Source: CAD feature listing. Evaluate the final solid. Frame: model axes, mm. A direction names the side the tool comes from. Round coordinates to 2 decimals unless told otherwise and drop trailing zeros. Loops run counter-clockwise (first coordinate to the right, second up) from the corner with the lowest first, then second, coordinate; pieces in that order, holes last. Notation, with made-up numbers: M -33,-2.75 L -4,-2.75 A24 ccw -4,10.25 Z; hole C 27.5,50.5 d6. An arc over 180 degrees is marked long. One line per item, written item: value.
from build123d import *

# Parameters (mm, degrees)
F0_R     = 3.175
F0_W     = 0.7229064099
F0_H     = 4.7706251523
F1_DEPTH = 3.048


with BuildPart() as f1:
    # F0 (on Front) → F1 (new body)
    with BuildSketch(Plane.XZ):
        with BuildLine():
            ThreePointArc((-9.4502929642, 115.490625), (-0.596483242, 104.7936951058), (9.525, 114.3))
            ThreePointArc((9.525, 114.3), (9.5063048942, 114.896483242), (9.4502929642, 115.490625))
            ThreePointArc((9.4502929642, 115.490625), (0, 123.825), (-9.4502929642, 115.490625))
        make_face()
        with Locations((0, 114.3)):
            Circle(F0_R, mode=Mode.SUBTRACT)
        with BuildLine():
            ThreePointArc((9.4502929642, 115.490625), (9.5063048942, 114.896483242), (9.525, 114.3))
            ThreePointArc((9.525, 114.3), (-0.596483242, 104.7936951058), (-9.4502929642, 115.490625))
            Line((-9.4502929642, 115.490625), (-15.7504882737, 65.484375))
            ThreePointArc((-15.7504882737, 65.484375), (0, 79.375), (15.7504882737, 65.484375))
            Line((15.7504882737, 65.484375), (9.4502929642, 115.490625))
        make_face()
        with Locations((-3.175, 100.0252)):
            Circle(F0_R, mode=Mode.SUBTRACT)
        with BuildLine():
            ThreePointArc((15.875, 63.5), (15.8438414904, 64.4941387366), (15.7504882737, 65.484375))
            ThreePointArc((15.7504882737, 65.484375), (0, 79.375), (-15.7504882737, 65.484375))
            ThreePointArc((-15.7504882737, 65.484375), (-15.8737438155, 63.6997054867), (-15.7954255641, 61.9125))
            ThreePointArc((-15.7954255641, 61.9125), (0, 47.625), (15.7954255641, 61.9125))
            ThreePointArc((15.7954255641, 61.9125), (15.8550939106, 62.7052534459), (15.875, 63.5))
        make_face()
        with Locations((0, 63.5)):
            Circle(F0_R, mode=Mode.SUBTRACT)
        with BuildLine():
            ThreePointArc((15.7954255641, 61.9125), (0, 47.625), (-15.7954255641, 61.9125))
            Line((-15.7954255641, 61.9125), (-9.4772553384, -0.9525))
            ThreePointArc((-9.4772553384, -0.9525), (-0.4768479324, 9.5130563464), (9.525, 0))
            ThreePointArc((9.525, 0), (6.8544082857, -6.6138273378), (0.3401785714, -9.5189234444))
            Line((0.3401785714, -9.5189234444), (44.7334821429, -7.9324362036))
            ThreePointArc((44.7334821429, -7.9324362036), (36.5125, 0), (44.7334821429, 7.9324362036))
            Line((44.7334821429, 7.9324362036), (18.9676000005, 8.8532337108))
            ThreePointArc((18.9676000005, 8.8532337108), (13.2611998974, 11.5713591498), (11.3411865923, 17.5933818124))
            Line((11.3411865923, 17.5933818124), (15.7954255641, 61.9125))
        make_face()
        Polygon((-5.7888228126, 31.6815939556), (-6.5549086035, 31.6815939556), (-7.3474591762, 33.7054533268), (-9.8978284182, 33.7054533268), (-10.6806288082, 31.6815939556), (-11.43, 31.6815939556), (-8.9144528394, 38.0721423349), (-8.2918340239, 38.0721423349), align=None, mode=Mode.SUBTRACT)
        with BuildLine():
            Line((-1.0349122593, 31.6815939556), (-1.7578186693, 31.6815939556))
            Line((-1.7578186693, 31.6815939556), (-1.7578186693, 34.7682232513))
            add(Edge.make_bspline(
                [(-1.7578186693, 34.7682232513), (-1.7578186693, 35.3504484524), (-2.0231629296, 35.6380788447)],
                knots=[0, 0, 0, 1, 1, 1], degree=2))
            add(Edge.make_bspline(
                [(-2.0231629296, 35.6380788447), (-2.2885071899, 35.9257092371), (-2.8554106751, 35.9257092371)],
                knots=[0, 0, 0, 1, 1, 1], degree=2))
            add(Edge.make_bspline(
                [(-2.8554106751, 35.9257092371), (-3.6033889837, 35.9257092371), (-3.9516097977, 35.5210766512)],
                knots=[0, 0, 0, 1, 1, 1], degree=2))
            add(Edge.make_bspline(
                [(-3.9516097977, 35.5210766512), (-4.2998306117, 35.1164440653), (-4.2998306117, 34.184605167)],
                knots=[0, 0, 0, 1, 1, 1], degree=2))
            Line((-4.2998306117, 34.184605167), (-4.2998306117, 31.6815939556))
            Line((-4.2998306117, 31.6815939556), (-5.0227370217, 31.6815939556))
            Line((-5.0227370217, 31.6815939556), (-5.0227370217, 36.452219108))
            Line((-5.0227370217, 36.452219108), (-4.4349402876, 36.452219108))
            Line((-4.4349402876, 36.452219108), (-4.3179380941, 35.7989568608))
            Line((-4.3179380941, 35.7989568608), (-4.2831160127, 35.7989568608))
            add(Edge.make_bspline(
                [(-4.2831160127, 35.7989568608), (-4.0602546917, 36.1513563246), (-3.6598007555, 36.3456635389)],
                knots=[0, 0, 0, 1, 1, 1], degree=2))
            add(Edge.make_bspline(
                [(-3.6598007555, 36.3456635389), (-3.2593468194, 36.5399707531), (-2.76765903, 36.5399707531)],
                knots=[0, 0, 0, 1, 1, 1], degree=2))
            add(Edge.make_bspline(
                [(-2.76765903, 36.5399707531), (-1.9054642944, 36.5399707531), (-1.4701882769, 36.1241951011)],
                knots=[0, 0, 0, 1, 1, 1], degree=2))
            add(Edge.make_bspline(
                [(-1.4701882769, 36.1241951011), (-1.0349122593, 35.7084194492), (-1.0349122593, 34.7932951499)],
                knots=[0, 0, 0, 1, 1, 1], degree=2))
            Line((-1.0349122593, 34.7932951499), (-1.0349122593, 31.6815939556))
        make_face(mode=Mode.SUBTRACT)
        with Locations((0.8099616135, 34.0669065318)):
            Rectangle(F0_W, F0_H, mode=Mode.SUBTRACT)
        with BuildLine():
            add(Edge.make_bspline(
                [(0.5090988301, 37.3812722398), (0.3872215452, 37.5010601999), (0.3872215452, 37.7448147697)],
                knots=[0, 0, 0, 1, 1, 1], degree=2))
            add(Edge.make_bspline(
                [(0.3872215452, 37.7448147697), (0.3872215452, 37.9927479893), (0.5090988301, 38.1083572995)],
                knots=[0, 0, 0, 1, 1, 1], degree=2))
            add(Edge.make_bspline(
                [(0.5090988301, 38.1083572995), (0.630976115, 38.2239666098), (0.8148367049, 38.2239666098)],
                knots=[0, 0, 0, 1, 1, 1], degree=2))
            add(Edge.make_bspline(
                [(0.8148367049, 38.2239666098), (0.9889471119, 38.2239666098), (1.1150030466, 38.1062679747)],
                knots=[0, 0, 0, 1, 1, 1], degree=2))
            add(Edge.make_bspline(
                [(1.1150030466, 38.1062679747), (1.2410589812, 37.9885693395), (1.2410589812, 37.7448147697)],
                knots=[0, 0, 0, 1, 1, 1], degree=2))
            add(Edge.make_bspline(
                [(1.2410589812, 37.7448147697), (1.2410589812, 37.5010601999), (1.1150030466, 37.3812722398)],
                knots=[0, 0, 0, 1, 1, 1], degree=2))
            add(Edge.make_bspline(
                [(1.1150030466, 37.3812722398), (0.9889471119, 37.2614842798), (0.8148367049, 37.2614842798)],
                knots=[0, 0, 0, 1, 1, 1], degree=2))
            add(Edge.make_bspline(
                [(0.8148367049, 37.2614842798), (0.630976115, 37.2614842798), (0.5090988301, 37.3812722398)],
                knots=[0, 0, 0, 1, 1, 1], degree=2))
        make_face(mode=Mode.SUBTRACT)
        with BuildLine():
            Line((3.3833134292, 34.1233183037), (3.4181355106, 34.1233183037))
            add(Edge.make_bspline(
                [(3.4181355106, 34.1233183037), (3.6047818669, 34.3893590056), (3.9878247624, 34.8197599318)],
                knots=[0, 0, 0, 1, 1, 1], degree=2))
            Line((3.9878247624, 34.8197599318), (5.5283536437, 36.452219108))
            Line((5.5283536437, 36.452219108), (6.3863697295, 36.452219108))
            Line((6.3863697295, 36.452219108), (4.4530477699, 34.4200024372))
            Line((4.4530477699, 34.4200024372), (6.5214794053, 31.6815939556))
            Line((6.5214794053, 31.6815939556), (5.6467487204, 31.6815939556))
            Line((5.6467487204, 31.6815939556), (3.9613599805, 33.9366719474))
            Line((3.9613599805, 33.9366719474), (3.4181355106, 33.4658774068))
            Line((3.4181355106, 33.4658774068), (3.4181355106, 31.6815939556))
            Line((3.4181355106, 31.6815939556), (2.7035864002, 31.6815939556))
            Line((2.7035864002, 31.6815939556), (2.7035864002, 38.4551852303))
            Line((2.7035864002, 38.4551852303), (3.4181355106, 38.4551852303))
            Line((3.4181355106, 38.4551852303), (3.4181355106, 34.8629393127))
            add(Edge.make_bspline(
                [(3.4181355106, 34.8629393127), (3.4181355106, 34.6247562759), (3.3833134292, 34.1233183037)],
                knots=[0, 0, 0, 1, 1, 1], degree=2))
        make_face(mode=Mode.SUBTRACT)
        with BuildLine():
            Line((10.8519534487, 31.6815939556), (10.3156933951, 31.6815939556))
            Line((10.3156933951, 31.6815939556), (10.1722264197, 32.3613209846))
            Line((10.1722264197, 32.3613209846), (10.1374043383, 32.3613209846))
            add(Edge.make_bspline(
                [(10.1374043383, 32.3613209846), (9.7808262247, 31.9128125762), (9.426337436, 31.7533274433)],
                knots=[0, 0, 0, 1, 1, 1], degree=2))
            add(Edge.make_bspline(
                [(9.426337436, 31.7533274433), (9.0718486473, 31.5938423105), (8.5397672435, 31.5938423105)],
                knots=[0, 0, 0, 1, 1, 1], degree=2))
            add(Edge.make_bspline(
                [(8.5397672435, 31.5938423105), (7.8307896661, 31.5938423105), (7.4282464051, 31.9601706069)],
                knots=[0, 0, 0, 1, 1, 1], degree=2))
            add(Edge.make_bspline(
                [(7.4282464051, 31.9601706069), (7.025703144, 32.3264989032), (7.025703144, 33.0006543992)],
                knots=[0, 0, 0, 1, 1, 1], degree=2))
            add(Edge.make_bspline(
                [(7.025703144, 33.0006543992), (7.025703144, 34.4450743359), (9.336496466, 34.5147184987)],
                knots=[0, 0, 0, 1, 1, 1], degree=2))
            Line((9.336496466, 34.5147184987), (10.1457616378, 34.5411832805))
            Line((10.1457616378, 34.5411832805), (10.1457616378, 34.8378674141))
            add(Edge.make_bspline(
                [(10.1457616378, 34.8378674141), (10.1457616378, 35.3991993663), (9.9047928345, 35.6666329515)],
                knots=[0, 0, 0, 1, 1, 1], degree=2))
            add(Edge.make_bspline(
                [(9.9047928345, 35.6666329515), (9.6638240312, 35.9340665367), (9.1317426273, 35.9340665367)],
                knots=[0, 0, 0, 1, 1, 1], degree=2))
            add(Edge.make_bspline(
                [(9.1317426273, 35.9340665367), (8.5355885937, 35.9340665367), (7.7834316354, 35.5691311236)],
                knots=[0, 0, 0, 1, 1, 1], degree=2))
            Line((7.7834316354, 35.5691311236), (7.5605703144, 36.1221057763))
            add(Edge.make_bspline(
                [(7.5605703144, 36.1221057763), (7.9129697782, 36.3129307824), (8.3329240799, 36.4215756763)],
                knots=[0, 0, 0, 1, 1, 1], degree=2))
            add(Edge.make_bspline(
                [(8.3329240799, 36.4215756763), (8.7528783817, 36.5302205703), (9.1763148915, 36.5302205703)],
                knots=[0, 0, 0, 1, 1, 1], degree=2))
            add(Edge.make_bspline(
                [(9.1763148915, 36.5302205703), (10.0287594443, 36.5302205703), (10.4403564465, 36.1520527663)],
                knots=[0, 0, 0, 1, 1, 1], degree=2))
            add(Edge.make_bspline(
                [(10.4403564465, 36.1520527663), (10.8519534487, 35.7738849622), (10.8519534487, 34.9381550085)],
                knots=[0, 0, 0, 1, 1, 1], degree=2))
            Line((10.8519534487, 34.9381550085), (10.8519534487, 31.6815939556))
        make_face(mode=Mode.SUBTRACT)
        with BuildLine():
            ThreePointArc((9.525, 0), (-0.4768479324, 9.5130563464), (-9.4772553384, -0.9525))
            ThreePointArc((-9.4772553384, -0.9525), (-6.2623833816, -7.1769199091), (0.3401785714, -9.5189234444))
            ThreePointArc((0.3401785714, -9.5189234444), (6.8544082857, -6.6138273378), (9.525, 0))
        make_face()
        Circle(F0_R, mode=Mode.SUBTRACT)
        with BuildLine():
            ThreePointArc((44.7334821429, 7.9324362036), (36.5125, 0), (44.7334821429, -7.9324362036))
            ThreePointArc((44.7334821429, -7.9324362036), (50.1620069047, -5.5115227815), (52.3875, 0))
            ThreePointArc((52.3875, 0), (50.1620069047, 5.5115227815), (44.7334821429, 7.9324362036))
        make_face()
        with Locations((44.45, 0)):
            Circle(F0_R, mode=Mode.SUBTRACT)
    extrude(amount=F1_DEPTH)


solid = f1.part
1. Section query B-B (y = -1.25). Count the separate pieces of the cut face and the enclosed holes in it, and give its area (3 significant figures).
Report:
separate pieces: 1
enclosed holes: 11
area: 3,730 mm2
2. Ray query, line 1 (Z direction, x = 5, y = -1.05); line 2 (Z direction, x = -8.5, y = -1.3); line 3 (X direction, y = -2.4, z = 50). Return the intervals inside material, ascending. Write a range as [from, to].
Report:
line 1: z = [-9.35, 32.55], [33.7, 34.99], [35.89, 122.41]
line 2: z = [-4.3, 33.71], [38.07, 118.6]
line 3: x = [-14.6, 14.6]
3. Section query C-C (z = 40). Return the cut outline in (x, y).
Report:
outline: M -13.59,-3.05 L 13.59,-3.05 L 13.59,0 L -13.59,0 Z
4. Pull-direction query (X, two-part tool) for faces 3 (the face through (2.704, -2, 35)), 4 (the face through (3, -3.048, 43)), 5 (the face through (13.321, -1.503, 11.503)), 6 (the face through (0.193, -1.503, 123.823)); classes: released by +X, released by -X, zero draft, split by the parting line, or undercut.
Report:
face 3: undercut
face 4: zero draft
face 5: released by +X
face 6: split by the parting line
5. Reachability of faces 1 (the face through (-5.023, -2, 34)), 2 (the face through (3, 0, 43)) from +Z, -Z, +X, -X, +Y, -Y: full face, straight path, thin tool, end or side. Return the list, or none.
Report:
face 1: +Y, -Y
face 2: +Z, -Z, +X, -X, +Y
6. Section query D-D (x = 21). Return the cut outline in (y, z).
Report:
outline: M -3.05,-8.78 L 0,-8.78 L 0,8.78 L -3.05,8.78 Z
7. Section query A-A (z = 102). Return the cut outline in (x, y).
Report:
outline: M -11.15,-3.05 L -5.66,-3.05 L -5.66,0 L -11.15,0 Z; M -0.69,-3.05 L 11.15,-3.05 L 11.15,0 L -0.69,0 Z
8. Pin query (flat end, axial travel): pin 1 (4 mm diameter, centred on x = 0, z = 0, fed in from +Y); pin 2 (8.5 mm diameter, centred on x = -3.18, z = 100.03, fed in from -Y); pin 3 (0.5 mm diameter, centred on x = -8.5, y = -1.5, fed in from -Z); pin 4 (0.6 mm diameter, centred on x = -5, y = -2, fed in from +Z). Return the tip coordinate at first contact, or that it passes through.
Report:
pin 1: passes through
pin 2: stops at y = -3.05
pin 3: stops at z = -4.76
pin 4: stops at z = 122.58
